Design review of the part built by this model. Coordinates are the model's own, in mm. Face numbers are marked on the shaded views. A direction names the side the tool comes from. Coordinates: 2 decimals unless noted, no trailing zeros. Order: outer loops, then holes, each group sorted by start corner. A loop starts at its lowest first (then second) coordinate and runs counter-clockwise, first axis right, second up. Notation, with made-up numbers: (-9, 83.25) -> (0, 83.25) arc R34 cw to (0, 114.25) -> close; hole circle Ø6 at (20, 20.25). An arc over 180 degrees is marked (long way). Use a Markdown table: item, result. Add a question column.
Q1. Add section B-B (x = -40). State the section outline as (y, z) points.
Q2. Insertion check: pin 1 (4 mm diameter, centred on y = 5, z = 100, fed in from -X); pin 2 (3 mm diameter, centred on y = 5, z = 175, fed in from +X); pin 3 (4 mm diameter, centred on y = 5, z = 100, fed in from +X); pin 4 (4.5 mm diameter, centred on y = 5, z = 175, fed in from -X). Each pin has a flat end and moves straight along its axis. Give the tip position at first contact, or say it passes through.
Q3. Wall thickness on probe 1 along Z at (x, y) = (-67.85, 5); probe 2 along X at (y, z) = (11.5, 135); probe 3 along Y at (x, z) = (-68, 175): over which ranges is each line inside the solid? List them lowest first.
Q4. Machinability: for the marked faces 1 and 2, which of the approach directions +Z, -Z, +X, -X, +Y, -Y give a long, thin tool a straight path to every point of the face, cutting with its end or side? Answer none if there is none.
Q5. Add section A-A (y = 12.5). State the section outline as (x, z) points.
Q6. The part is to be moulded in two halves that separate along X. For the marked faces 3, 4 and 5, say which applies: pulls with the +X half, pulls with the -X half, needs draft (parallel to the pull), parting line crosses it, or undercut.
Autodesk Inventor part; units mm, degrees
ref_plane "YZ Plane" through (0, 0, 0) normal (1, 0, 0) x (0, 1, 0)
ref_plane "XZ Plane" through (0, 0, 0) normal (0, 1, 0) x (-1, 0, 0)
ref_plane "XY Plane" through (0, 0, 0) normal (0, 0, 1) x (1, 0, 0)
sketch "Skizze1" plane through (0, 0, 0) normal (0, 0, 1) x (1, 0, 0)
  line L0 (-99.5698, 0) -> (99.5698, 0)
  line L1 (0, -20.7243) -> (0, 124.3456)
  line L2 (67.5, 0) -> (67.5, 100)
  line L3 (67.5, 100) -> (-67.5, 100)
  line L4 (-67.5, 100) -> (-67.5, 0)
  line L5 (67.5, 0) -> (70.5, 0)
  line L6 (70.5, 0) -> (70.5, 100)
  line L7 (67.5, 103) -> (-67.5, 103)
  line L8 (-70.5, 100) -> (-70.5, 0)
  line L9 (-70.5, 0) -> (-67.5, 0)
  arc A0 (-67.5, 103) -> (-70.5, 100) centre (-67.5, 100) ccw
  arc A1 (70.5, 100) -> (67.5, 103) centre (67.5, 100) ccw
  point P0 (0, 0)
  dimension "d0" = 135
  dimension "d1" = 3
  dimension "d2" = 100
  dimension "d3" = 3
  dimension "d4" = 3
extrude "Extrusion1" add sketch "Skizze1" along normal blind 200 contours L8 A0 L7 L1 L3 L4 L0 | L2 L3 L1 L7 A1 L6 L0
sketch "Skizze2" plane through (70.5, 0, 0) normal (1, 0, 0) x (0, 0, -1)
  line L0 (-200, 100) -> (-200, 0)
  line L1 (0, 0) -> (-200, 0)
  line L2 (0, 0) -> (0, 100)
  line L3 (0, 100) -> (-200, 100)
  line L4 (-200, 5) -> (0, 5)
  line L5 (-100, 100) -> (-100, 0)
  point P0 (-175, 5)
  point P1 (-25, 5)
  point P2 (-100, 5)
  dimension "d7" = 5
  dimension "d8" = 25
  dimension "d9" = 25
hole "Bohrung1" at (70.5, 5, 175) at (70.5, 5, 25) at (70.5, 5, 100) direction (-1, 0, 0) diameter 3.4 end through all countersink diameter 6.9 countersink angle 90
sketch "Skizze3" plane through (-70.5, 0, 0) normal (-1, 0, 0) x (0, 0, 1)
  circle A0 centre (100, 5) radius 1.7
  circle A1 centre (25, 5) radius 1.7
  circle A2 centre (175, 5) radius 1.7
  point P0 (25, 5)
  point P1 (100, 5)
  point P2 (175, 5)
hole "Bohrung2" at (-70.5, 5, 25) at (-70.5, 5, 100) at (-70.5, 5, 175) direction (1, 0, 0) diameter 3.4 end through all countersink diameter 6.9 countersink angle 90
properties part number "13_0204_059"
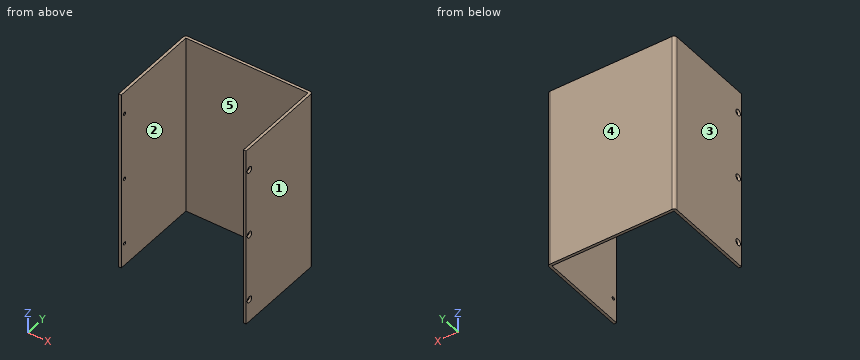
Established:
| question | item | result |
|---|---|---|
| 1 | outline | (100, 0) -> (103, 0) -> (103, 200) -> (100, 200) -> close |
| 2 | pin 1 | x = -69.05 |
| 2 | pin 2 | through |
| 2 | pin 3 | x = 69.05 |
| 2 | pin 4 | x = -69.3 |
| 3 | probe 1 | 0 to 23.3, 26.7 to 98.3, 101.7 to 173.3, 176.7 to 200 |
| 3 | probe 2 | -70.5 to -67.5, 67.5 to 70.5 |
| 3 | probe 3 | 0 to 3.3, 6.7 to 102.96 |
| 4 | face 1 | +Z, -Z, +X, +Y, -Y |
| 4 | face 2 | +Z, -Z, -Y |
| 5 | outline | (-70.5, 0) -> (-67.5, 0) -> (-67.5, 200) -> (-70.5, 200) -> close; (67.5, 0) -> (70.5, 0) -> (70.5, 200) -> (67.5, 200) -> close |
| 6 | face 3 | pulls with the -X half |
| 6 | face 4 | needs draft |
| 6 | face 5 | undercut |
